from build123d import *

# Parameters (mm, degrees)
SKETCH2_R               = 9
BOSS_EXTRUDE1_DEPTH     = 381
SKETCH3_R               = 9.5
BOSS_EXTRUDE2_DEPTH     = 1.5875
SKETCH4_R               = 3.175
CUT_EXTRUDE1_DEPTH      = 10.5
CUT_EXTRUDE1_DEPTH_BACK = 10.5


with BuildPart() as part:
    # Sketch2 → Boss-Extrude1 (new body)
    with BuildSketch(Plane(origin=(0, 0, 0), x_dir=(1, 0, 0), z_dir=(0, 1, 0))):
        Circle(SKETCH2_R)
    extrude(amount=BOSS_EXTRUDE1_DEPTH)

    # Sketch3 → Boss-Extrude2 (add)
    with BuildSketch(Plane.XZ):
        Circle(SKETCH3_R)
    extrude(amount=-BOSS_EXTRUDE2_DEPTH)

    # Sketch4 → Cut-Extrude1 (cut, two sides)
    with BuildSketch(Plane(origin=(0, 0, 0), x_dir=(0, 0, -1), z_dir=(1, 0, 0))) as cut_extrude1_sk:
        with Locations((0, 372)):
            Circle(SKETCH4_R)
    extrude(amount=CUT_EXTRUDE1_DEPTH, mode=Mode.SUBTRACT)
    extrude(cut_extrude1_sk.sketch, amount=-CUT_EXTRUDE1_DEPTH_BACK, mode=Mode.SUBTRACT)


solid = part.part
Work out the finished part from the listing and answer in its coordinate system (mm). A direction names the side the tool comes from. Coordinates: 2 decimals unless noted, no trailing zeros. Loops run counter-clockwise (first coordinate to the right, second up) from the corner with the lowest first, then second, coordinate; pieces in that order, holes last. Notation, with made-up numbers: M 43,28.5 L 89,28.5 A19 ccw 89,48.5 Z; hole C 58,-20.5 d9. An arc over 180 degrees is marked long. Answer in a Markdown table with one row per item. Add a question column.
1. Flat-ended cylindrical pins translate along their axes: P1, Ø1.5, axis at x = -7.5, y = 169, coming from the +Z side; P2, Ø10, axis at x = -6.5, y = 157, coming from the +Z side; P3, Ø4, axis at y = 372, z = 0, coming from the -X side; P4, Ø4, axis at y = 49, z = 7.5, coming from the -X side. Find the tip coordinate at first contact, or state that the pin passes through.
2. Find section D-D, the plane y = 224.5. Write down the section's boundary in (x, z), then the cut area to 3 significant figures.
3. A tool of negligible diameter and unlimited length cuts with its end or side. For faces 1 (the flat face through (-6, 1.588, -7)), 2 (the cylindrical face through (4.38, 0.78, -8.43)), from which of +Z, -Z, +X, -X, +Y, -Y can it reach the whole face along a straight path? Write none if from no direction.
4. Find section A-A, the plane z = 0. Write down the section's boundary in (x, y) (1 decimal).
5. Consider L1, parallel to Y at x = -4.25, z = 0 (3 decimals); L2, parallel to Y at x = 3.25, z = -0.5; L3, parallel to Z at x = 0.5, y = 75. Determine where each line is inside the solid, lowest interval first.
6. Find section C-C, the plane y = 372. Write down the section's boundary in (x, z) (3 decimals), then the cut area to 3 significant figures.
Reported:
| question | item | result |
|---|---|---|
| 1 | P1 | stops at z = 5.95 |
| 1 | P2 | stops at z = 8.87 |
| 1 | P3 | passes through |
| 1 | P4 | stops at x = -7.12 |
| 2 | outline | C 0,0 d18 |
| 2 | area | 254 mm^2 |
| 3 | face 1 | +Y |
| 3 | face 2 | +Y, -Y |
| 4 | outline | M -9.5,0 L 9.5,0 L 9.5,1.6 L 9,1.6 L 9,368.8 L -9,368.8 L -9,1.6 L -9.5,1.6 Z; M -9,375.2 L 9,375.2 L 9,381 L -9,381 Z |
| 5 | L1 | y = 0 to 368.825, 375.175 to 381 |
| 5 | L2 | y = 0 to 368.86, 375.14 to 381 |
| 5 | L3 | z = -8.99 to 8.99 |
| 6 | outline | M -8.421,-3.175 A9 ccw 8.421,-3.175 Z; M -8.421,3.175 L 8.421,3.175 A9 ccw Z |
| 6 | area | 143 mm^2 |
